from build123d import *

# Parameters (mm, degrees)
F0_W     = 89.622184
F0_H     = 92.715051
F1_DEPTH = 88.079302
F2_R     = 24.954129
F3_DEPTH = 179.480271


with BuildPart() as f1:
    # F0 (on Front) → F1 (new body)
    with BuildSketch(Plane.XZ):
        with Locations((-1.479607, 12.499084)):
            Rectangle(F0_W, F0_H)
    extrude(amount=F1_DEPTH)

    # F2 (on face) → F3 (join)
    with BuildSketch(Plane.XZ.offset(88.079302)):
        Circle(F2_R)
    extrude(amount=-F3_DEPTH)


solid = f1.part
Can you work these out from the model? Positions are in its coordinate system, mm. A direction names the side the tool comes from. Give positions to 0.01 mm unless a question says otherwise; leave off trailing zeros. Write each loop counter-clockwise with the first axis right and the second up, starting at its lowest first coordinate (ties: lowest second). Pieces come first, ordered by that corner, then holes. Notation, with made-up numbers: M -21.75,42 L -15.75,42 A21 ccw -15.75,53 Z; hole C -32.5,45 d11. An arc over 180 degrees is marked long. Answer in a Markdown table with one row per item. Add a question column.
Item 1: For pin 1 Ø8 at (x, y) = (0.5, 42) entering from +Z; pin 2 Ø1 at (x, z) = (-27.5, -3) entering from +Y; pin 3 Ø6 at (x, y) = (-12, 36.5) entering from +Z, each with a flat end and sliding along its axis, tell me the tip position at first contact or that it passes through.
Item 2: Imagine slicing it at C-C, the plane z = 35.5. Write out the boundary of the cut face in (x, y), plus the area to 3 significant figures.
Item 3: Imagine slicing it at B-B, the plane z = -11. Write out the boundary of the cut face in (x, y).
Item 4: Imagine slicing it at A-A, the plane x = 0. Write out the boundary of the cut face in (y, z).
Item 5: On a 3-axis mill with a long thin cutter (end or side, diameter ignored), from which of +Z, -Z, +X, -X, +Y, -Y can I reach the whole of each face in a straight line? I mean faces 1 (the flat face through (-2, -43, -33.858)), 2 (the cylindrical face through (23.8, 45.1, 7.5)). Say none if no direction works.
Item 6: Please list where these lines run through material, in increasing order: L1, parallel to Y at x = 37.5, z = 35; L2, parallel to X at y = 40.5, z = 1; L3, parallel to X at y = 45, z = 10.
Evaluation:
| question | item | result |
|---|---|---|
| 1 | pin 1 | stops at z = 24.95 |
| 1 | pin 2 | stops at y = 0 |
| 1 | pin 3 | stops at z = 23.27 |
| 2 | outline | M -46.29,-88.08 L 43.33,-88.08 L 43.33,0 L -46.29,0 Z |
| 2 | area | 7,890 mm² |
| 3 | outline | M -46.29,-88.08 L 43.33,-88.08 L 43.33,0 L 22.4,0 L 22.4,91.4 L -22.4,91.4 L -22.4,0 L -46.29,0 Z |
| 4 | outline | M -88.08,-33.86 L 0,-33.86 L 0,-24.95 L 91.4,-24.95 L 91.4,24.95 L 0,24.95 L 0,58.86 L -88.08,58.86 Z |
| 5 | face 1 | -Z, +X, -X, +Y, -Y |
| 5 | face 2 | +Y |
| 6 | L1 | y = -88.08 to 0 |
| 6 | L2 | x = -24.93 to 24.93 |
| 6 | L3 | x = -22.86 to 22.86 |
